from build123d import *

# Parameters (mm, degrees)
SKETCH1_W           = 100
SKETCH1_H           = 220
SKETCH1_R           = 2.05
SKETCH1_R_2         = 1.6
BOSS_EXTRUDE1_DEPTH = 5
CUT_EXTRUDE1_DEPTH  = 10


with BuildPart() as part:
    # Sketch1 → Boss-Extrude1 (new body)
    with BuildSketch(Plane(origin=(0, 0, 0), x_dir=(1, 0, 0), z_dir=(0, 1, 0))):
        Rectangle(SKETCH1_W, SKETCH1_H)
        with Locations(Location((-44, 104, 0), (0, 0, 270))):
            Circle(SKETCH1_R, mode=Mode.SUBTRACT)
        with Locations(Location((-34.072831353, 76.618821882, 0), (0, 0, 270))):
            Circle(SKETCH1_R_2, mode=Mode.SUBTRACT)
        with Locations(Location((-0.472623192, 95.381178118, 0), (0, 0, 270))):
            Circle(SKETCH1_R_2, mode=Mode.SUBTRACT)
        with Locations(Location((-21.170351419, 67.157003264, 0), (0, 0, 270))):
            Circle(SKETCH1_R_2, mode=Mode.SUBTRACT)
        with Locations(Location((-13.375103126, 104.842996736, 0), (0, 0, 270))):
            Circle(SKETCH1_R_2, mode=Mode.SUBTRACT)
        with Locations(Location((-0.472623192, -95.381178118, 0), (0, 0, 90))):
            Circle(SKETCH1_R_2, mode=Mode.SUBTRACT)
        with Locations(Location((-21.170351419, -67.157003264, 0), (0, 0, 90))):
            Circle(SKETCH1_R_2, mode=Mode.SUBTRACT)
        with Locations(Location((-34.072831353, -76.618821882, 0), (0, 0, 90))):
            Circle(SKETCH1_R_2, mode=Mode.SUBTRACT)
        with Locations(Location((-44, -104, 0), (0, 0, 90))):
            Circle(SKETCH1_R, mode=Mode.SUBTRACT)
        with Locations(Location((-13.375103126, -104.842996736, 0), (0, 0, 90))):
            Circle(SKETCH1_R_2, mode=Mode.SUBTRACT)
        with BuildLine():
            Line((39.45, -35), (39.45, 35))
            ThreePointArc((39.45, 35), (42, 37.55), (44.55, 35))
            Line((44.55, 35), (44.55, -35))
            ThreePointArc((44.55, -35), (42, -37.55), (39.45, -35))
        make_face(mode=Mode.SUBTRACT)
        with BuildLine():
            Line((-39.45, -35), (-39.45, 35))
            ThreePointArc((-39.45, 35), (-42, 37.55), (-44.55, 35))
            Line((-44.55, 35), (-44.55, -35))
            ThreePointArc((-44.55, -35), (-42, -37.55), (-39.45, -35))
        make_face(mode=Mode.SUBTRACT)
    extrude(amount=BOSS_EXTRUDE1_DEPTH)

    # Sketch2 → Cut-Extrude1 (cut)
    with BuildSketch(Plane(origin=(0, 5, 0), x_dir=(1, 0, 0), z_dir=(0, 1, 0))):
        with BuildLine():
            Line((4.46621247, 110), (50, 110))
            Line((50, 110), (50, 44.175543471))
            ThreePointArc((50, 44.175543471), (40.575458137, 59.361991758), (26.838854749, 70.796847608))
            ThreePointArc((26.838854749, 70.796847608), (10.452936433, 87.431092849), (4.46621247, 110))
        make_face()
        with BuildLine():
            Line((50, -44.175543471), (50, -110))
            Line((50, -110), (4.46621247, -110))
            ThreePointArc((4.46621247, -110), (10.452936433, -87.431092849), (26.838854749, -70.796847608))
            ThreePointArc((26.838854749, -70.796847608), (40.575458137, -59.361991758), (50, -44.175543471))
        make_face()
    extrude(amount=-CUT_EXTRUDE1_DEPTH, mode=Mode.SUBTRACT)


solid = part.part
Verification items for the finished model (mm, model axes). A direction names the side the tool comes from. Round coordinates to 2 decimals unless told otherwise and drop trailing zeros. Order: outer loops, then holes, each group sorted by start corner. A loop starts at its lowest first (then second) coordinate and runs counter-clockwise, first axis right, second up.
1. Section check A-A on z = -16.5. Record the cut outline in (x, y).
Final values:
outline: (-50, 0) - (-44.55, 0) - (-44.55, 5) - (-50, 5) - close; (-39.45, 0) - (39.45, 0) - (39.45, 5) - (-39.45, 5) - close; (44.55, 0) - (50, 0) - (50, 5) - (44.55, 5) - close
2. Access from +Z, -Z, +X, -X, +Y, -Y to the whole of each face (thin tool, end or side, straight path). Record for faces 4 (the flat face through (-39.45, 2, 0)), 5 (the flat face through (-50, 2, 2)).
Final values:
face 4: +Y, -Y
face 5: +Z, -Z, -X, +Y, -Y
3. Thickness scan on L1, parallel to X at y = 1.85, z = 22.5; L2, parallel to X at y = 2.25, z = 104; L3, parallel to Z at x = -1.5, y = 0.9. Record the ranges inside material, lowest first.
Final values:
L1: x = -50 to -44.55, -39.45 to 39.45, 44.55 to 50
L2: x = -50 to -46.05, -41.95 to -14.74, -12.02 to 4.86
L3: z = -110 to -96.61, -94.15 to 94.15, 96.61 to 110
4. Section check D-D on x = 31.5. Record the cut outline in (y, z), then the cut area to 3 significant figures.
Final values:
outline: (0, -67.72) - (5, -67.72) - (5, 67.72) - (0, 67.72) - close
area: 677 mm2
5. Release check for a two-part mould opening along Z. For faces 1 (the flat face through (-12, 5, -2)), 2 (the cylindrical face through (42.06, 2.46, 37.55)), 3 (the flat face through (-23, 2, 110)) record: +Z half, -Z half, draft (parallel to the pull), parting line (faces both ways), or undercut.
Final values:
face 1: draft
face 2: undercut
face 3: +Z half
6. Section check C-C on y = 3.85. State how many separate pieces and enclosed holes the cut face has, then the cut area to 3 significant figures.
Final values:
separate pieces: 1
enclosed holes: 12
area: 17,600 mm2
7. Go/stop test with a flat-tipped pin: P1, Ø2.5, axis at x = -21.17, z = -67.16, coming from the +Y side. Record where the tip stops, or that it passes through.
Final values:
P1: passes through
8. Section check B-B on x = 42. Record the cut outline in (y, z).
Final values:
outline: (0, -57.66) - (5, -57.66) - (5, -37.55) - (0, -37.55) - close; (0, 37.55) - (5, 37.55) - (5, 57.66) - (0, 57.66) - close
